```python
from build123d import *

# Parameters (mm, degrees)
F1_DEPTH = 248.92
F2_W     = 33.02
F2_H     = 243.84
F3_DEPTH = 48.26


with BuildPart() as f1:
    # F0 (on Top) → F1 (new body)
    with BuildSketch(Plane.XY):
        with BuildLine():
            ThreePointArc((-19.05, 0), (0, 19.05), (19.05, 0))
            Line((19.05, 0), (19.05, 50.8))
            Line((19.05, 50.8), (-19.05, 50.8))
            Line((-19.05, 50.8), (-19.05, 0))
        make_face()
        with BuildLine():
            Line((-19.05, 0), (19.05, 0))
            ThreePointArc((19.05, 0), (0, 19.05), (-19.05, 0))
        make_face()
        with BuildLine():
            ThreePointArc((-19.05, 0), (0, -19.05), (19.05, 0))
            Line((19.05, 0), (-19.05, 0))
        make_face()
    extrude(amount=F1_DEPTH)

    # F2 (on face) → F3 (cut)
    with BuildSketch(Plane(origin=(0, 50.8, 0), x_dir=(-1, 0, 0), z_dir=(0, 1, 0))):
        with Locations((0, 124.46)):
            Rectangle(F2_W, F2_H)
    extrude(amount=-F3_DEPTH, mode=Mode.SUBTRACT)


solid = f1.part
```
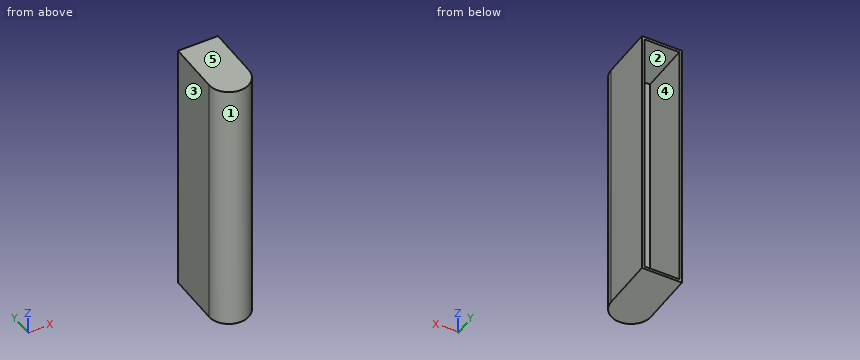
Model file for the job. Use its own axes, mm. Face numbers are marked on the shaded views. A direction names the side the tool comes from. Give positions to 0.01 mm unless a question says otherwise; leave off trailing zeros. Write each loop counter-clockwise with the first axis right and the second up, starting at its lowest first coordinate (ties: lowest second). Pieces come first, ordered by that corner, then holes. Notation, with made-up numbers: M 28.25,-19.5 L 69.25,-19.5 A32 ccw 69.25,18.5 Z; hole C 18,58 d8. An arc over 180 degrees is marked long. Use a Markdown table: item, result.
1) Pull direction Z, two halves, no side cores. Call the marked faces 3, 4 and 5: +Z half, -Z half, draft (parallel to the pull), parting line (faces both ways), or undercut.
Responses:
| item | result |
|---|---|
| face 3 | draft |
| face 4 | undercut |
| face 5 | +Z half |
2) Drill centre lines: line 1 (Z direction, x = 11, y = 3); line 2 (X direction, y = 41, z = 57.5); line 3 (Y direction, x = 1, z = 36.5). Where is each one in solid material? Low to high. Write a range as from..to.
Responses:
| item | result |
|---|---|
| line 1 | z = 0..2.54, 246.38..248.92 |
| line 2 | x = -19.05..-16.51, 16.51..19.05 |
| line 3 | y = -19.02..2.54 |
3) Cut at D-D (y = -13.5). List the corners of the cut face in (x, z), and give its area (3 significant figures).
Responses:
| item | result |
|---|---|
| outline | M -13.44,0 L 13.44,0 L 13.44,248.92 L -13.44,248.92 Z |
| area | 6,690 mm2 |
4) Cut at C-C (z = 65). List the corners of the cut face in (x, y).
Responses:
| item | result |
|---|---|
| outline | M -19.05,0 A19.05 ccw 19.05,0 L 19.05,50.8 L 16.51,50.8 L 16.51,2.54 L -16.51,2.54 L -16.51,50.8 L -19.05,50.8 Z |
5) Pin check, flat tips, straight feed: pin 1 (3 mm diameter, centred on y = -6.5, z = 155.5, fed in from +X); pin 2 (2 mm diameter, centred on x = -11.5, z = 152.5, fed in from +Y). Stop position of each tip, or through.
Responses:
| item | result |
|---|---|
| pin 1 | stops at x = 18.38 |
| pin 2 | stops at y = 2.54 |
6) Cut at A-A (x = 0). List the corners of the cut face in (y, z).
Responses:
| item | result |
|---|---|
| outline | M -19.05,0 L 50.8,0 L 50.8,2.54 L 2.54,2.54 L 2.54,246.38 L 50.8,246.38 L 50.8,248.92 L -19.05,248.92 Z |
7) Tool access for the marked faces 1 and 2: list every direction of +Z, -Z, +X, -X, +Y, -Y with a clear straight run to the whole face (end or side of a thin tool).
Responses:
| item | result |
|---|---|
| face 1 | +Z, -Z, -Y |
| face 2 | +Y |
8) Cut at B-B (y = 45.5). List the corners of the cut face in (x, z), and give its area (3 significant figures).
Responses:
| item | result |
|---|---|
| outline | M -19.05,0 L 19.05,0 L 19.05,248.92 L -19.05,248.92 Z; hole M -16.51,2.54 L 16.51,2.54 L 16.51,246.38 L -16.51,246.38 Z |
| area | 1,430 mm2 |
